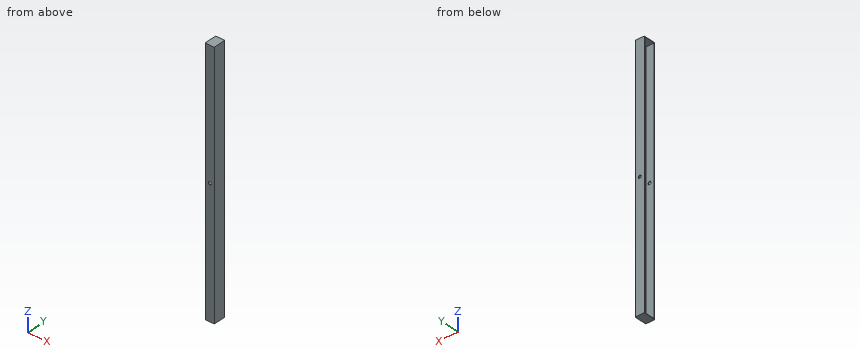
```python
from build123d import *

# Parameters (mm, degrees)
BOSS_EXTRUDE1_DEPTH = 533.4
SKETCH2_R           = 3.175
CUT_EXTRUDE1_DEPTH  = 381
SKETCH4_W           = 19.05
SKETCH4_H           = 25.4
BOSS_EXTRUDE3_DEPTH = 1.016
SKETCH5_W           = 19.05
SKETCH5_H           = 25.4
BOSS_EXTRUDE4_DEPTH = 1.016


with BuildPart() as part:
    # Sketch1 → Boss-Extrude1 (new body)
    with BuildSketch(Plane.XY):
        Polygon((0, 0), (17.4625, 0), (17.4625, -22.225), (0, -22.225), (0, -23.8125), (12.7, -23.8125), (19.05, -23.8125), (19.05, 0), (19.05, 1.5875), (0, 1.5875), align=None)
    extrude(amount=BOSS_EXTRUDE1_DEPTH)

    # Sketch2 → Cut-Extrude1 (cut)
    with BuildSketch(Plane(origin=(0, 1.5875, 0), x_dir=(1, 0, 0), z_dir=(0, 1, 0))):
        with Locations((9.525, -266.7)):
            Circle(SKETCH2_R)
    extrude(amount=-CUT_EXTRUDE1_DEPTH, mode=Mode.SUBTRACT)

    # Sketch4 → Boss-Extrude3 (add)
    with BuildSketch(Plane(origin=(0, 0, 0), x_dir=(-1, 0, 0), z_dir=(0, 0, -1))):
        with Locations((-9.525, -11.1125)):
            Rectangle(SKETCH4_W, SKETCH4_H)
    extrude(amount=BOSS_EXTRUDE3_DEPTH)

    # Sketch5 → Boss-Extrude4 (add)
    with BuildSketch(Plane.XY.offset(533.4)):
        with Locations((9.525, -11.1125)):
            Rectangle(SKETCH5_W, SKETCH5_H)
    extrude(amount=BOSS_EXTRUDE4_DEPTH)


solid = part.part
```
The model under review builds one solid part; all positions refer to its coordinate system, in mm. Round coordinates to 2 decimals unless told otherwise and drop trailing zeros. Write each loop counter-clockwise with the first axis right and the second up, starting at its lowest first coordinate (ties: lowest second). Pieces come first, ordered by that corner, then holes. Notation, with made-up numbers: (-14, 10) -> (23, 10) arc R21 cw to (23, 38) -> close; hole circle Ø4 at (5.25, 14). An arc over 180 degrees is marked (long way). Use CSV: the item, a comma, the result in double quotes.
Q1. Consider section A-A (x = 3). Give the boundary of the cut face in (y, z) (1 decimal), then the cut area to 3 significant figures.
Checks:
outline,"(-23.8, -1) -> (1.6, -1) -> (1.6, 534.4) -> (-23.8, 534.4) -> close; hole (-22.2, 0) -> (0, 0) -> (0, 533.4) -> (-22.2, 533.4) -> close"
area,"1,750 mm²"
Q2. For pin 1 Ø5 at (x, z) = (9.525, 266.7) entering from +Y; pin 2 Ø4 at (y, z) = (-9.5, 341) entering from -X, all flat-tipped, find the tip position at first contact; note any pin that passes through.
Checks:
pin 1,"through"
pin 2,"x = 17.46"
Q3. Consider section C-C (y = -14). Give the boundary of the cut face in (x, z).
Checks:
outline,"(0, -1.02) -> (19.05, -1.02) -> (19.05, 534.42) -> (0, 534.42) -> (0, 533.4) -> (17.46, 533.4) -> (17.46, 0) -> (0, 0) -> close"
Q4. To check wall thickness, follow probe 1 along Y at (x, z) = (3.75, 176.5) (1 decimal); probe 2 along Z at (x, y) = (16.25, -13.5); probe 3 along X at (y, z) = (-22.6, 266.7). State the ranges of each line that lie inside material, in increasing order. Write a range as [from, to].
Checks:
probe 1,"[-23.8, -22.2], [0, 1.6]"
probe 2,"[-1.02, 0], [533.4, 534.42]"
probe 3,"[0, 6.35], [12.7, 19.05]"
